Geometry check sheet. Reference: the model listing, model coordinates, mm. Face numbers are marked on the shaded views. Coordinates: 2 decimals unless noted, no trailing zeros. Loops run counter-clockwise (first coordinate to the right, second up) from the corner with the lowest first, then second, coordinate; pieces in that order, holes last.
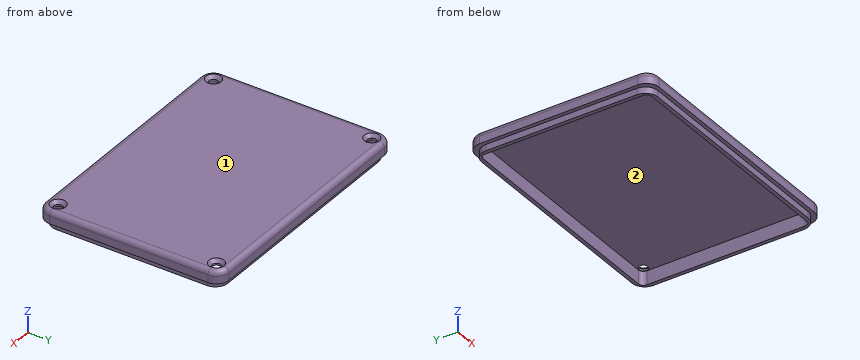
from build123d import *

# Parameters (mm, degrees)
F0_W           = 101
F0_H           = 73
F0_W_2         = 98
F0_H_2         = 70
F0_W_3         = 95
F0_H_3         = 67
F1_DEPTH       = 5
F2_DEPTH       = 3
F3_DEPTH       = 2.5
F4_R           = 2
F5_T1_DEPTH    = 2.5
F5_T3_DEPTH    = 5
F5_T6_ANGLE    = 90
F5_T8_ANGLE    = 90
F5_T10_ANGLE   = 90
F5_T12_ANGLE   = 90
F7_D           = 3.5
F7_DEPTH       = 6
F7_CSINK_D     = 6
F7_CSINK_ANGLE = 90
F7_TIP         = 1.0515060833


# Not quite as in the source:
# - a fillet or chamfer that OpenCascade refuses, or shapes differently, is made with other operations: its cross-section is extruded or revolved along the edge and cut away or added
# - a feature names something its author has since deleted; it is built from what else it names


with BuildPart() as f1:
    # F0 (on Top) → F1 (new body)
    with BuildSketch(Plane.XY):
        Rectangle(F0_W, F0_H)
        Rectangle(F0_W_2, F0_H_2, mode=Mode.SUBTRACT)
        Rectangle(F0_W_2, F0_H_2)
        Rectangle(F0_W_3, F0_H_3, mode=Mode.SUBTRACT)
        Rectangle(F0_W_3, F0_H_3)
    extrude(amount=F1_DEPTH)

    # F0 (on Top) → F2 (cut)
    with BuildSketch(Plane.XY):
        Rectangle(F0_W_3, F0_H_3)
    extrude(amount=F2_DEPTH, mode=Mode.SUBTRACT)

    # F0 (on Top) → F3 (join)
    with BuildSketch(Plane.XY):
        Rectangle(F0_W_2, F0_H_2)
        Rectangle(F0_W_3, F0_H_3, mode=Mode.SUBTRACT)
    extrude(amount=-F3_DEPTH)

    # F4
    f4_edges = [f1.edges().sort_by_distance(p)[0] for p in [
        (-47.5, -33.5, 0.25),
        (-47.5, 33.5, 0.25),
        (47.5, 33.5, 0.25),
        (47.5, -33.5, 0.25),
        (0, -36.5, 5),
        (50.5, 0, 5),
        (-50.5, 0, 5),
        (0, 36.5, 5),
    ]]
    fillet(f4_edges, radius=F4_R)

    # F5: fillet of radius 5 on 8 edges, made by hand

    # F5_s2 → F5_t1 (cut)
    with BuildSketch(Plane.XY.offset(-2.5)):
        with BuildLine():
            ThreePointArc((-44, -35), (-47.5355339059, -33.5355339059), (-49, -30))
            Line((-49, -30), (-49.1, -30))
            Line((-49.1, -30), (-49.1, -35.1))
            Line((-49.1, -35.1), (-44, -35.1))
            Line((-44, -35.1), (-44, -35))
        make_face()
        with BuildLine():
            ThreePointArc((44, -35), (47.5355339059, -33.5355339059), (49, -30))
            Line((49, -30), (49.1, -30))
            Line((49.1, -30), (49.1, -35.1))
            Line((49.1, -35.1), (44, -35.1))
            Line((44, -35.1), (44, -35))
        make_face()
        with BuildLine():
            ThreePointArc((49, 30), (47.5355339059, 33.5355339059), (44, 35))
            Line((44, 35), (44, 35.1))
            Line((44, 35.1), (49.1, 35.1))
            Line((49.1, 35.1), (49.1, 30))
            Line((49.1, 30), (49, 30))
        make_face()
        with BuildLine():
            ThreePointArc((-44, 35), (-47.5355339059, 33.5355339059), (-49, 30))
            Line((-49, 30), (-49.1, 30))
            Line((-49.1, 30), (-49.1, 35.1))
            Line((-49.1, 35.1), (-44, 35.1))
            Line((-44, 35.1), (-44, 35))
        make_face()
    extrude(amount=F5_T1_DEPTH, mode=Mode.SUBTRACT)

    # F5_s4 → F5_t3 (cut)
    with BuildSketch(Plane.XY):
        with BuildLine():
            ThreePointArc((-50.5, -31.5), (-49.0355339059, -35.0355339059), (-45.5, -36.5))
            Line((-45.5, -36.5), (-45.5, -36.6))
            Line((-45.5, -36.6), (-50.6, -36.6))
            Line((-50.6, -36.6), (-50.6, -31.5))
            Line((-50.6, -31.5), (-50.5, -31.5))
        make_face()
        with BuildLine():
            ThreePointArc((50.5, -31.5), (49.0355339059, -35.0355339059), (45.5, -36.5))
            Line((45.5, -36.5), (45.5, -36.6))
            Line((45.5, -36.6), (50.6, -36.6))
            Line((50.6, -36.6), (50.6, -31.5))
            Line((50.6, -31.5), (50.5, -31.5))
        make_face()
        with BuildLine():
            ThreePointArc((45.5, 36.5), (49.0355339059, 35.0355339059), (50.5, 31.5))
            Line((50.5, 31.5), (50.6, 31.5))
            Line((50.6, 31.5), (50.6, 36.6))
            Line((50.6, 36.6), (45.5, 36.6))
            Line((45.5, 36.6), (45.5, 36.5))
        make_face()
        with BuildLine():
            ThreePointArc((-45.5, 36.5), (-49.0355339059, 35.0355339059), (-50.5, 31.5))
            Line((-50.5, 31.5), (-50.6, 31.5))
            Line((-50.6, 31.5), (-50.6, 36.6))
            Line((-50.6, 36.6), (-45.5, 36.6))
            Line((-45.5, 36.6), (-45.5, 36.5))
        make_face()
    extrude(amount=F5_T3_DEPTH, mode=Mode.SUBTRACT)

    # F5_s5 → F5_t6 (revolve, cut)
    with BuildSketch(Plane.YZ.offset(-45.5)):
        with BuildLine():
            ThreePointArc((34.5, 5), (35.9142135624, 4.4142135624), (36.5, 3))
            Line((36.5, 3), (36.5, 5))
            Line((36.5, 5), (34.5, 5))
        make_face()
    revolve(axis=Axis((-45.5, 31.5, 5), (0, 0, 1)), revolution_arc=F5_T6_ANGLE, mode=Mode.SUBTRACT)

    # F5_s7 → F5_t8 (revolve, cut)
    with BuildSketch(Plane.XZ.offset(-31.5)):
        with BuildLine():
            ThreePointArc((48.5, 5), (49.9142135624, 4.4142135624), (50.5, 3))
            Line((50.5, 3), (50.5, 5))
            Line((50.5, 5), (48.5, 5))
        make_face()
    revolve(axis=Axis((45.5, 31.5, 5), (0, 0, 1)), revolution_arc=F5_T8_ANGLE, mode=Mode.SUBTRACT)

    # F5_s9 → F5_t10 (revolve, cut)
    with BuildSketch(Plane.YZ.offset(45.5)):
        with BuildLine():
            ThreePointArc((-34.5, 5), (-35.9142135624, 4.4142135624), (-36.5, 3))
            Line((-36.5, 3), (-36.5, 5))
            Line((-36.5, 5), (-34.5, 5))
        make_face()
    revolve(axis=Axis((45.5, -31.5, 5), (0, 0, 1)), revolution_arc=F5_T10_ANGLE, mode=Mode.SUBTRACT)

    # F5_s11 → F5_t12 (revolve, cut)
    with BuildSketch(Plane.XZ.offset(31.5)):
        with BuildLine():
            ThreePointArc((-48.5, 5), (-49.9142135624, 4.4142135624), (-50.5, 3))
            Line((-50.5, 3), (-50.5, 5))
            Line((-50.5, 5), (-48.5, 5))
        make_face()
    revolve(axis=Axis((-45.5, -31.5, 5), (0, 0, 1)), revolution_arc=F5_T12_ANGLE, mode=Mode.SUBTRACT)

    # F7
    with Locations(Plane.XY.offset(5)):
        with Locations((45.5, -31.5), (-45.5, -31.5), (-45.5, 31.5), (45.5, 31.5)):
            CounterSinkHole(F7_D / 2, F7_CSINK_D / 2, depth=F7_DEPTH, counter_sink_angle=F7_CSINK_ANGLE)
            with Locations((0, 0, -(F7_DEPTH + F7_TIP / 2))):  # 118° drill point
                Cone(0, F7_D / 2, F7_TIP, mode=Mode.SUBTRACT)


solid = f1.part
(1) Gauge pin test, flat ends, axial feed: pin 1 Ø12 at (x, y) = (-13, -1.5) entering from -Z; pin 2 Ø1.2 at (x, z) = (0.5, -1.5) entering from +Y; pin 3 Ø3 at (x, y) = (45.5, 31.5) entering from +Z; pin 4 Ø1.2 at (y, z) = (-5.5, -1.5) entering from -X. Record the tip position at first contact, or that the pin passes through.
Findings:
pin 1: stops at z = 3
pin 2: stops at y = 35
pin 3: passes through
pin 4: stops at x = -49
(2) Sectioned sample at B-B on y = -24.5. Record the cut outline in (x, z), and give its area (3 significant figures).
Findings:
outline: (-50.5, 0) - (-49, 0) - (-49, -2.5) - (-47.5, -2.5) - (-47.5, 3) - (47.5, 3) - (47.5, -2.5) - (49, -2.5) - (49, 0) - (50.5, 0) - (50.5, 3) arc R2 ccw to (48.5, 5) - (-48.5, 5) arc R2 ccw to (-50.5, 3) - close
area: 226 mm2
(3) Sectioned sample at A-A on z = -1.5. Record the cut outline in (x, y), and give its area (3 significant figures).
Findings:
outline: (-49, -30) arc R5 ccw to (-44, -35) - (44, -35) arc R5 ccw to (49, -30) - (49, 30) arc R5 ccw to (44, 35) - (-44, 35) arc R5 ccw to (-49, 30) - close; hole (-47.5, -31.5) arc R2 ccw to (-45.5, -33.5) - (45.5, -33.5) arc R2 ccw to (47.5, -31.5) - (47.5, 31.5) arc R2 ccw to (45.5, 33.5) - (-45.5, 33.5) arc R2 ccw to (-47.5, 31.5) - close
area: 477 mm2
(4) Sectioned sample at C-C on x = -9. Record the cut outline in (y, z).
Findings:
outline: (-36.5, 0) - (-35, 0) - (-35, -2.5) - (-33.5, -2.5) - (-33.5, 3) - (33.5, 3) - (33.5, -2.5) - (35, -2.5) - (35, 0) - (36.5, 0) - (36.5, 3) arc R2 ccw to (34.5, 5) - (-34.5, 5) arc R2 ccw to (-36.5, 3) - close
(5) Draft check along Y on the marked faces 1 and 2. Enter one of: +Y half, -Y half, draft (parallel to the pull), parting line (faces both ways), or undercut.
Findings:
face 1: draft
face 2: undercut
(6) Scan lines: L1, parallel to X at y = -31.5, z = 3.25; L2, parallel to X at y = -13, z = -0.25; L3, parallel to Y at x = -22, z = 1. Record each from-to range of solid material in increasing order.
Findings:
L1: x = -50.48 to -47.25, -43.75 to 43.75, 47.25 to 50.48
L2: x = -49 to -47.5, 47.5 to 49
L3: y = -36.5 to -33.5, 33.5 to 36.5
